from build123d import *

# Parameters (mm, degrees)
SZKIC2_W                             = 555
SZKIC2_H                             = 265
ODGI_CIE_BAZOWE1_DEPTH               = 1
ODGI_CIE_KRAW_DZI1_STRIP_W           = 5.4732
ODGI_CIE_KRAW_DZI1_STRIP_H           = 1
ODGI_CIE_KRAW_DZI1_STRIP_CUT_DEPTH   = 265
ODGI_CIE_KRAW_DZI1_STRIP_2_W         = 5.4732
ODGI_CIE_KRAW_DZI1_STRIP_2_H         = 1
ODGI_CIE_KRAW_DZI1_STRIP_CUT_2_DEPTH = 265
ODGI_CIE_KRAW_DZI1_DEPTH             = 265
ODGI_CIE_KRAW_DZI1_BEND_DEPTH        = 265
WYTNIJ_WYCI_GNI_CIE3_DEPTH           = 574.436352179
ZAOKR_GLENIE2_R                      = 10
SZKIC16_R                            = 2
WYTNIJ_WYCI_GNI_CIE4_DEPTH           = 10
WYTNIJ_WYCI_GNI_CIE5_DEPTH           = 10
ZAOKR_GLENIE3_R                      = 10


# Sheet-metal steps are written as plain solids
with BuildPart() as part:
    # Szkic2 → Odgięcie bazowe1 (new body)
    with BuildSketch(Plane(origin=(0, 0, 0), x_dir=(1, 0, 0), z_dir=(0, 1, 0))):
        Rectangle(SZKIC2_W, SZKIC2_H)
    extrude(amount=-ODGI_CIE_BAZOWE1_DEPTH)

    # Odgięcie krawędzi1 strip (across the edge) → Odgięcie krawędzi1 strip cut (cut)
    with BuildSketch(Plane(origin=(-277.5, -1, 132.5), x_dir=(1, 0, 0), z_dir=(0, 0, -1))):
        with Locations((-2, -0.5)):
            Rectangle(ODGI_CIE_KRAW_DZI1_STRIP_W, ODGI_CIE_KRAW_DZI1_STRIP_H)
    extrude(amount=ODGI_CIE_KRAW_DZI1_STRIP_CUT_DEPTH, mode=Mode.SUBTRACT)

    # Odgięcie krawędzi1 strip 2 (across the edge) → Odgięcie krawędzi1 strip cut 2 (cut)
    with BuildSketch(Plane(origin=(277.5, -1, -132.5), x_dir=(-1, 0, 0), z_dir=(0, 0, 1))):
        with Locations((-2, -0.5)):
            Rectangle(ODGI_CIE_KRAW_DZI1_STRIP_2_W, ODGI_CIE_KRAW_DZI1_STRIP_2_H)
    extrude(amount=ODGI_CIE_KRAW_DZI1_STRIP_CUT_2_DEPTH, mode=Mode.SUBTRACT)

    # Odgięcie krawędzi1 section (across the edge) → Odgięcie krawędzi1 (add)
    with BuildSketch(Plane(origin=(-277.5, -1, 132.5), x_dir=(1, 0, 0), z_dir=(0, 0, -1))):
        with BuildLine():
            Line((-1, 0.7366), (-1, 31))
            Line((-1, 31), (0, 31))
            Line((0, 31), (0, 0.7366))
            ThreePointArc((0, 0.7366), (0.215745145, 0.215745145), (0.7366, 0))
            Line((0.7366, 0), (0.7366, -1))
            ThreePointArc((0.7366, -1), (-0.491361636, -0.491361636), (-1, 0.7366))
        make_face()
    extrude(amount=ODGI_CIE_KRAW_DZI1_DEPTH)

    # Odgięcie krawędzi1 section 2 (across the edge) → Odgięcie krawędzi1 bend (add)
    with BuildSketch(Plane(origin=(277.5, -1, -132.5), x_dir=(-1, 0, 0), z_dir=(0, 0, 1))):
        with BuildLine():
            Line((-1, 0.7366), (-1, 31))
            Line((-1, 31), (0, 31))
            Line((0, 31), (0, 0.7366))
            ThreePointArc((0, 0.7366), (0.215745145, 0.215745145), (0.7366, 0))
            Line((0.7366, 0), (0.7366, -1))
            ThreePointArc((0.7366, -1), (-0.491361636, -0.491361636), (-1, 0.7366))
        make_face()
    extrude(amount=ODGI_CIE_KRAW_DZI1_BEND_DEPTH)

    # Szkic15 → Wytnij-wyciągnięcie3 (cut, through all)
    with BuildSketch(Plane(origin=(278.5, 0, 0), x_dir=(0, 0, -1), z_dir=(1, 0, 0))):
        with BuildLine():
            Line((-97.75, -22), (-97.75, -27))
            ThreePointArc((-97.75, -27), (-100.25, -29.5), (-102.75, -27))
            Line((-102.75, -27), (-102.75, -22))
            ThreePointArc((-102.75, -22), (-100.25, -19.5), (-97.75, -22))
        make_face()
        with BuildLine():
            Line((-22.75, -22), (-22.75, -27))
            ThreePointArc((-22.75, -27), (-20.25, -29.5), (-17.75, -27))
            Line((-17.75, -27), (-17.75, -22))
            ThreePointArc((-17.75, -22), (-20.25, -19.5), (-22.75, -22))
        make_face()
        with BuildLine():
            Line((57.25, -22), (57.25, -27))
            ThreePointArc((57.25, -27), (59.75, -29.5), (62.25, -27))
            Line((62.25, -27), (62.25, -22))
            ThreePointArc((62.25, -22), (59.75, -19.5), (57.25, -22))
        make_face()
    extrude(amount=-WYTNIJ_WYCI_GNI_CIE3_DEPTH, mode=Mode.SUBTRACT)

    # Zaokrąglenie2
    zaokr_glenie2_edges = [part.edges().sort_by_distance(p)[0] for p in [
        (-278, -32, 132.5),
        (-278, -32, -132.5),
        (278, -32, -132.5),
        (278, -32, 132.5),
    ]]
    fillet(zaokr_glenie2_edges, radius=ZAOKR_GLENIE2_R)

    # Szkic16 → Wytnij-wyciągnięcie4 (cut)
    with BuildSketch(Plane(origin=(0, 0, 0), x_dir=(1, 0, 0), z_dir=(0, 1, 0))):
        with Locations(Location((-258.25, -125.25, 0), (0, 0, 270))):
            Circle(SZKIC16_R)
        with Locations(Location((-186.75, -125.25, 0), (0, 0, 270))):
            Circle(SZKIC16_R)
        with Locations(Location((-258.25, 76.25, 0), (0, 0, 270))):
            Circle(SZKIC16_R)
        with Locations(Location((-186.75, 76.25, 0), (0, 0, 270))):
            Circle(SZKIC16_R)
        with Locations(Location((-169.25, 76.25, 0), (0, 0, 270))):
            Circle(SZKIC16_R)
        with Locations(Location((-97.75, 76.25, 0), (0, 0, 270))):
            Circle(SZKIC16_R)
        with Locations(Location((-169.25, -125.25, 0), (0, 0, 270))):
            Circle(SZKIC16_R)
        with Locations(Location((-97.75, -125.25, 0), (0, 0, 270))):
            Circle(SZKIC16_R)
        with Locations(Location((-80.25, 76.25, 0), (0, 0, 270))):
            Circle(SZKIC16_R)
        with Locations(Location((-8.75, 76.25, 0), (0, 0, 270))):
            Circle(SZKIC16_R)
        with Locations(Location((-80.25, -125.25, 0), (0, 0, 270))):
            Circle(SZKIC16_R)
        with Locations(Location((-8.75, -125.25, 0), (0, 0, 270))):
            Circle(SZKIC16_R)
        with Locations(Location((8.75, 76.25, 0), (0, 0, 270))):
            Circle(SZKIC16_R)
        with Locations(Location((80.25, 76.25, 0), (0, 0, 270))):
            Circle(SZKIC16_R)
        with Locations(Location((8.75, -125.25, 0), (0, 0, 270))):
            Circle(SZKIC16_R)
        with Locations(Location((80.25, -125.25, 0), (0, 0, 270))):
            Circle(SZKIC16_R)
        with Locations(Location((97.75, 76.25, 0), (0, 0, 270))):
            Circle(SZKIC16_R)
        with Locations(Location((169.25, 76.25, 0), (0, 0, 270))):
            Circle(SZKIC16_R)
        with Locations(Location((97.75, -125.25, 0), (0, 0, 270))):
            Circle(SZKIC16_R)
        with Locations(Location((169.25, -125.25, 0), (0, 0, 270))):
            Circle(SZKIC16_R)
        with Locations(Location((186.75, 76.25, 0), (0, 0, 270))):
            Circle(SZKIC16_R)
        with Locations(Location((258.25, 76.25, 0), (0, 0, 270))):
            Circle(SZKIC16_R)
        with Locations(Location((186.75, -125.25, 0), (0, 0, 270))):
            Circle(SZKIC16_R)
        with Locations(Location((258.25, -125.25, 0), (0, 0, 270))):
            Circle(SZKIC16_R)
    extrude(amount=-WYTNIJ_WYCI_GNI_CIE4_DEPTH, mode=Mode.SUBTRACT)

    # Szkic17 → Wytnij-wyciągnięcie5 (cut)
    with BuildSketch(Plane(origin=(0, 0, 0), x_dir=(1, 0, 0), z_dir=(0, 1, 0))):
        with BuildLine():
            Line((15, 102.5), (-15, 102.5))
            ThreePointArc((-15, 102.5), (-22.071067812, 105.428932188), (-25, 112.5))
            Line((-25, 112.5), (-25, 132.5))
            Line((-25, 132.5), (25, 132.5))
            Line((25, 132.5), (25, 112.5))
            ThreePointArc((25, 112.5), (22.071067812, 105.428932188), (15, 102.5))
        make_face()
        with BuildLine():
            Line((155, 132.5), (205, 132.5))
            Line((205, 132.5), (205, 112.5))
            ThreePointArc((205, 112.5), (202.071067812, 105.428932188), (195, 102.5))
            Line((195, 102.5), (165, 102.5))
            ThreePointArc((165, 102.5), (157.928932188, 105.428932188), (155, 112.5))
            Line((155, 112.5), (155, 132.5))
        make_face()
        with BuildLine():
            Line((-155, 112.5), (-155, 132.5))
            Line((-155, 132.5), (-205, 132.5))
            Line((-205, 132.5), (-205, 112.5))
            ThreePointArc((-205, 112.5), (-202.071067812, 105.428932188), (-195, 102.5))
            Line((-195, 102.5), (-165, 102.5))
            ThreePointArc((-165, 102.5), (-157.928932188, 105.428932188), (-155, 112.5))
        make_face()
    extrude(amount=-WYTNIJ_WYCI_GNI_CIE5_DEPTH, mode=Mode.SUBTRACT)

    # Zaokrąglenie3
    zaokr_glenie3_edges = [part.edges().sort_by_distance(p)[0] for p in [
        (25, -0.5, -132.5),
        (-25, -0.5, -132.5),
        (-155, -0.5, -132.5),
        (-205, -0.5, -132.5),
        (205, -0.5, -132.5),
        (155, -0.5, -132.5),
    ]]
    fillet(zaokr_glenie3_edges, radius=ZAOKR_GLENIE3_R)


solid = part.part
Work out the finished part from the listing and answer in its coordinate system (mm). A direction names the side the tool comes from. Coordinates: 2 decimals unless noted, no trailing zeros. Loops run counter-clockwise (first coordinate to the right, second up) from the corner with the lowest first, then second, coordinate; pieces in that order, holes last. Notation, with made-up numbers: M 51.25,-2 L 85.25,-2 A7 cw 85.25,7 Z; hole C -25.75,16.25 d4. An arc over 180 degrees is marked long. Answer in a Markdown table with one row per item. Add a question column.
1. Flat-ended cylindrical pins translate along their axes: P1, Ø0.8, axis at x = 278, y = -25, coming from the -Z side; P2, Ø1.1, axis at x = -278, y = -24, coming from the -Z side; P3, Ø3.5, axis at x = -97.75, z = 125.25, coming from the -Y side; P4, Ø1.5, axis at x = -115.5, z = 50, coming from the -Y side. Find the tip coordinate at first contact, or state that the pin passes through.
2. Find section A-A, the plane z = 10. Write down the section's boundary in (x, y), then the cut area to 3 significant figures.
3. Find section B-B, the plane x = -226. Write down the section's boundary in (y, z).
4. The mould has two halves that part along X. Classify faces 4 (the flat face through (-278.5, -17, 2)), 5 (the cylindrical face through (208.01, -0.51, -129.65)), 6 (the cylindrical face through (-277.99, -28.99, -129.65)): pulls with the +X half, pulls with the -X half, needs draft (parallel to the pull), parting line crosses it, or undercut.
5. Consider L1, parallel to Z at x = -258.25, y = -0.2; L2, parallel to X at y = -15.5, z = 53; L3, parallel to Y at x = 28, z = 58.5. Determine where each line is inside the solid, lowest interval first.
6. A tool of negligible diameter and unlimited length cuts with its end or side. For faces 1 (the cylindrical face through (-158.01, -0.49, -105.35)), 2 (the flat face through (-277.5, -17, 2)), 3 (the flat face through (-246.9, -0.5, -132.5)), from which of +Z, -Z, +X, -X, +Y, -Y can it reach the whole face along a straight path? Write none if from no direction.
Reported:
| question | item | result |
|---|---|---|
| 1 | P1 | stops at z = -132.16 |
| 1 | P2 | stops at z = -132.39 |
| 1 | P3 | passes through |
| 1 | P4 | stops at y = -1 |
| 2 | outline | M -278.5,-32 L -277.5,-32 L -277.5,-1.74 A0.74 cw -276.76,-1 L 276.76,-1 A0.74 cw 277.5,-1.74 L 277.5,-32 L 278.5,-32 L 278.5,-1.74 A1.74 ccw 276.76,0 L -276.76,0 A1.74 ccw -278.5,-1.74 Z |
| 2 | area | 618 mm^2 |
| 3 | outline | M -1,-132.5 L 0,-132.5 L 0,132.5 L -1,132.5 Z |
| 4 | face 4 | pulls with the -X half |
| 4 | face 5 | undercut |
| 4 | face 6 | needs draft |
| 5 | L1 | z = -132.5 to -78.25, -74.25 to 123.25, 127.25 to 132.5 |
| 5 | L2 | x = -278.5 to -277.5, 277.5 to 278.5 |
| 5 | L3 | y = -1 to 0 |
| 6 | face 1 | -Z, +Y, -Y |
| 6 | face 2 | +Z, -Z, -Y |
| 6 | face 3 | -Z, +X, -X, +Y, -Y |
